Input: part model. Units: mm. Frame: model coordinates. Face numbers are marked on the shaded views. A direction names the side the tool comes from. Coordinates: 2 decimals unless noted, no trailing zeros. Write each loop counter-clockwise with the first axis right and the second up, starting at its lowest first coordinate (ties: lowest second). Pieces come first, ordered by that corner, then holes. Notation, with made-up numbers: M -15,9.5 L 8,9.5 A29 cw 8,40.5 Z; hole C -40,74 d10. An arc over 180 degrees is marked long. Write each question's results on one line, items separated by ' | '. Start each with the question number.
1. Set-up query: the marked faces 1 and 2. Return all of +Z, -Z, +X, -X, +Y, -Y with unobstructed straight access to the full face (end or side cutting, diameter ignored); none if empty.
2. First-contact query: pin 1 (3 mm diameter, centred on x = -12.5, y = -40, fed in from +Z). Flat tip, straight axial feed; report the tip coordinate or a pass-through.
3. Section query C-C, the plane z = 1.5. Output: boundary loops of the cut face in (x, y), and give its area (3 significant figures).
4. Ray query, probe 1 along X at (y, z) = (-55, 4.75); probe 2 along Y at (x, z) = (7, 3); probe 3 along X at (y, z) = (-64.5, 2). Return the intervals inside material, ascending.
5. Section query D-D, the plane y = -55. Output: boundary loops of the cut face in (x, z), and give its area (3 significant figures).
6. Pull-direction query (Y, two-part tool) for the marked faces 3, 4 and 5; classes: +Y half, -Y half, draft (parallel to the pull), parting line (faces both ways), or undercut.
7. Section query B-B, the plane y = -44. Output: boundary loops of the cut face in (x, z), and give its area (3 significant figures).
8. Section query A-A, the plane x = 6. Output: boundary loops of the cut face in (y, z), and give its area (3 significant figures).
Autodesk Inventor part; units mm, degrees
ref_plane "YZ Plane" through (0, 0, 0) normal (1, 0, 0) x (0, 1, 0)
ref_plane "XZ Plane" through (0, 0, 0) normal (0, 1, 0) x (-1, 0, 0)
ref_plane "XY Plane" through (0, 0, 0) normal (0, 0, 1) x (1, 0, 0)
ref_plane "РабПлоскость1" through (0, 0, 0) normal (0, 0, 1) x (1, 0, 0)
sketch "Эскиз1" plane through (0, 0, 0) normal (0, 0, 1) x (1, 0, 0)
  line L0 (-20, -75) -> (20, -35) construction
  line L1 (20, -75) -> (-20, -35) construction
  line L2 (51, -62.7546) -> (51, 0.2454)
  line L3 (-51, 0.2454) -> (-51, -62.7546)
  line L4 (23.7454, -78.7454) -> (-23.7454, -78.7454)
  line L5 (-23.7454, -78.7454) -> (-23.7454, -31.2546)
  line L6 (-23.7454, -31.2546) -> (23.7454, -31.2546)
  line L7 (23.7454, -31.2546) -> (23.7454, -78.7454)
  line L8 (23.7454, -78.7454) -> (-23.7454, -31.2546) construction
  line L9 (-23.7454, -78.7454) -> (23.7454, -31.2546) construction
  point P0 (0, 0)
  point P1 (0, -55)
  point P2 (0, -55)
  dimension "d0" = 40
  dimension "d1" = 40
  dimension "d2" = 55
  dimension "d3" = 51
extrude "Выдавливание1" add sketch "Эскиз1" along normal blind 10
fillet "Сопряжение1" radius 2 4 edges at (-23.7454, -78.7454, 5) (23.7454, -78.7454, 5) (23.7454, -31.2546, 5) (-23.7454, -31.2546, 5)
sketch "Эскиз2" plane through (0, 0, 10) normal (0, 0, 1) x (1, 0, 0)
  line L0 (21.7454, -31.2546) -> (-21.7454, -31.2546)
  line L1 (0, -31.2546) -> (0, -78.7454)
  line L2 (-21.7454, -78.7454) -> (21.7454, -78.7454)
  line L3 (-23.7454, -33.2546) -> (-23.7454, -76.7454)
  line L4 (-23.7454, -55) -> (23.7454, -55)
  line L5 (23.7454, -76.7454) -> (23.7454, -33.2546)
  line L6 (0, -55) -> (-11.8725, -55)
  circle A0 centre (-11.8725, -55) radius 2
  circle A1 centre (11.8725, -55) radius 2
  point P0 (0, 0)
  dimension "d7" = 11.8725
  dimension "d8" = 4
extrude "Выдавливание2" cut sketch "Эскиз2" against normal blind 10
sketch "Эскиз3" plane through (0, 0, 10) normal (0, 0, 1) x (1, 0, 0)
  line L0 (-21.7454, -78.7454) -> (21.7454, -78.7454)
  line L1 (0, -78.7454) -> (0, -31.2546)
  line L2 (21.7454, -31.2546) -> (-21.7454, -31.2546)
  line L3 (-23.7454, -33.2546) -> (-23.7454, -76.7454)
  line L4 (-23.7454, -55) -> (23.7454, -55)
  line L5 (23.7454, -76.7454) -> (23.7454, -33.2546)
  line L6 (15, -74.9954) -> (-15, -74.9954)
  line L7 (-15, -74.9954) -> (-15, -62.4954)
  line L8 (-15, -62.4954) -> (15, -62.4954)
  line L9 (15, -62.4954) -> (15, -74.9954)
  line L10 (15, -74.9954) -> (-15, -62.4954) construction
  line L11 (-15, -74.9954) -> (15, -62.4954) construction
  line L12 (-21.7454, -78.7454) -> (21.7454, -78.7454)
  line L13 (15, -35.0046) -> (-15, -35.0046)
  line L14 (-15, -35.0046) -> (-15, -47.5046)
  line L15 (-15, -47.5046) -> (15, -47.5046)
  line L16 (15, -47.5046) -> (15, -35.0046)
  point P0 (0, 0)
  point P1 (0, -68.7454)
  dimension "d11" = 30
  dimension "d12" = 12.5
  dimension "d13" = 10
extrude "Выдавливание3" cut sketch "Эскиз3" against normal blind 10
properties part number "голова"
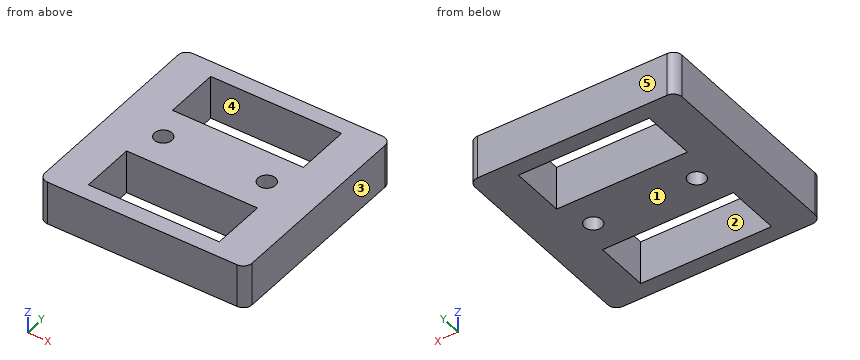
Answer:
1) face 1: -Z, +X, -X, +Y, -Y | face 2: +Z, -Z
2) pin 1: through
3) outline: M -23.75,-76.75 A2 ccw -21.75,-78.75 L 21.75,-78.75 A2 ccw 23.75,-76.75 L 23.75,-33.25 A2 ccw 21.75,-31.25 L -21.75,-31.25 A2 ccw -23.75,-33.25 Z; hole M -15,-75 L 15,-75 L 15,-62.5 L -15,-62.5 Z; hole M -15,-47.5 L 15,-47.5 L 15,-35 L -15,-35 Z; hole C -11.87,-55 d4; hole C 11.87,-55 d4 | area: 1,480 mm^2
4) probe 1: -23.75 to -13.87, -9.87 to 9.87, 13.87 to 23.75 | probe 2: -78.75 to -75, -62.5 to -47.5, -35 to -31.25 | probe 3: -23.75 to -15, 15 to 23.75
5) outline: M -23.75,0 L -13.87,0 L -13.87,10 L -23.75,10 Z; M -9.87,0 L 9.87,0 L 9.87,10 L -9.87,10 Z; M 13.87,0 L 23.75,0 L 23.75,10 L 13.87,10 Z | area: 395 mm^2
6) face 3: draft | face 4: undercut | face 5: +Y half
7) outline: M -23.75,0 L -15,0 L -15,10 L -23.75,10 Z; M 15,0 L 23.75,0 L 23.75,10 L 15,10 Z | area: 175 mm^2
8) outline: M -78.75,0 L -75,0 L -75,10 L -78.75,10 Z; M -62.5,0 L -47.5,0 L -47.5,10 L -62.5,10 Z; M -35,0 L -31.25,0 L -31.25,10 L -35,10 Z | area: 225 mm^2
